For this review, take the finished solid that the model builds, in its own axes (mm). A direction names the side the tool comes from. Give positions to 0.01 mm unless a question says otherwise; leave off trailing zeros. Write each loop counter-clockwise with the first axis right and the second up, starting at its lowest first coordinate (ties: lowest second). Pieces come first, ordered by that corner, then holes.
1) For P1, Ø3, axis at y = -1, z = -4, coming from the -X side; P2, Ø2.5, axis at x = -11.5, y = 0, coming from the +Z side; P3, Ø0.8, axis at x = -8.5, z = -2.5, coming from the -Y side, all flat-tipped, find the tip position at first contact; note any pin that passes through.
2) Draft analysis for pull direction X (two halves, no side actions). For faces 5 (the face through (-1.615, 2.389, 4.751)), 6 (the face through (-13, 0, -1)), 7 (the face through (-12, 0, 0.4)), state which applies: pulls with the +X half, pulls with the -X half, needs draft (parallel to the pull), parting line crosses it, or undercut.
3) Machinability: for faces 1 (the face through (-8.4, -0.8, 2.2)), 2 (the face through (-8.5, -1.6, 0)), 3 (the face through (6.385, 2.389, -3.249)), 4 (the face through (6.5, -1, 0)), which of the approach directions +Z, -Z, +X, -X, +Y, -Y give a long, thin tool a straight path to every point of the face, cutting with its end or side? Answer none if there is none.
4) We need section D-D on y = 2.5. Give the boundary of the cut face in (x, z).
5) Wall thickness on line 1 along Z through (x, y) = (5, -0.75); line 2 along X through (y, z) = (1, 2); line 3 along X through (y, z) = (-0.5, 1.75): over which ranges is each line inside the solid? List them lowest first.
6) We need section B-B on x = -2.5. Give the boundary of the cut face in (y, z), and give its area (3 significant figures).
7) We need section A-A on y = 0. Give the boundary of the cut face in (x, z).
8) We need section C-C on z = 4. Give the boundary of the cut face in (x, y), and give its area (3 significant figures).
Autodesk Inventor part; units mm, degrees
ref_plane "YZ Plane" through (0, 0, 0) normal (1, 0, 0) x (0, 1, 0)
ref_plane "XZ Plane" through (0, 0, 0) normal (0, 1, 0) x (-1, 0, 0)
ref_plane "XY Plane" through (0, 0, 0) normal (0, 0, 1) x (1, 0, 0)
sketch "Sketch1" plane through (0, 0, 0) normal (0, 0, 1) x (1, 0, 0)
  line L0 (8, 1.6) -> (-8, 1.6)
  line L1 (-8, 1.6) -> (-8, -4.8)
  line L2 (-8, -4.8) -> (0, -4.8)
  line L3 (8, -1.6) -> (8, 1.6)
  line L4 (0, -4.8) -> (0, -1.6)
  line L5 (0, -1.6) -> (8, -1.6)
  line L6 (-11.2, 0) -> (11.2, 0) construction
  line L7 (0, -6.08) -> (0, 2.88) construction
  point P0 (0, 1.6)
  point P1 (8, 0)
  dimension "d0" = 16
  dimension "d1" = 3.2
  dimension "d2" = 6.4
extrude "Extrusion1" add sketch "Sketch1" along normal mid plane 16
sketch "Sketch2" plane through (-8, 1.6, 8) normal (0, 1, 0) x (1, 0, 0)
  line L0 (4, 12) -> (12, 12) construction
  line L1 (12, 12) -> (12, 4) construction
  line L2 (12, 4) -> (4, 4) construction
  line L3 (4, 4) -> (4, 12) construction
  line L4 (-3.2, 8) -> (19.2, 8) construction
  line L5 (8, 19.2) -> (8, -3.2) construction
  circle A0 centre (4, 12) radius 2.5
  circle A1 centre (12, 12) radius 2.5
  circle A2 centre (12, 4) radius 2.5
  circle A3 centre (4, 4) radius 2.5
  point P0 (8, 12)
  point P1 (12, 8)
  dimension "d5" = 8
  dimension "d6" = 5
extrude "Extrusion2" add sketch "Sketch2" along normal blind 1.6
sketch "Sketch4" plane through (0, 0, 0) normal (0, 1, 0) x (-1, 0, 0)
  line L0 (8, -8) -> (8, 8) construction
  line L1 (14, 0) -> (7, 0) construction
  line L2 (8, 0) -> (8, -1.6)
  line L3 (8, -1.6) -> (9, -1.6)
  line L4 (9, -1.6) -> (9, -1.4)
  line L5 (9, -1.4) -> (12.2, -1.4)
  line L6 (12.2, -1.4) -> (12.2, -1.6)
  line L7 (12.2, -1.6) -> (13, -1.6)
  line L8 (13, -1.6) -> (13, 0)
  line L9 (13, 0) -> (8, 0)
  dimension "d9" = 2.8
  dimension "d11" = 3.2
  dimension "d12" = 5
  dimension "d13" = 3.2
  dimension "d14" = 0.8
revolve "Revolution1" add sketch "Sketch4" angle 360 about axis through (-13, 0, 0) along (1, 0, 0)
sketch "Sketch5" plane through (0, 0, 0) normal (0, 1, 0) x (-1, 0, 0)
  line L0 (9, 1.6) -> (9, -1.6)
  line L1 (8, -8) -> (8, 8)
  line L2 (9, -1.6) -> (8, -3.3321)
  line L3 (9, 1.6) -> (8, 3.3321)
  dimension "d16" = 30
extrude "Extrusion3" add sketch "Sketch5" along normal mid plane 1.6
sketch "Sketch6" plane through (0, 0, 0) normal (0, 1, 0) x (-1, 0, 0)
  line L0 (13, 1.6) -> (13, -1.6) construction
  line L1 (13, -0.4) -> (10.9, -0.4)
  arc A0 (10.9, 0.4) -> (10.9, -0.4) centre (10.9, 0) ccw
  line L2 (10.9, 0.4) -> (13, 0.4)
  line L3 (13, 0.4) -> (13, -0.4)
  point P0 (13, 0)
  dimension "d19" = 0.8
  dimension "d20" = 2.5
extrude "Extrusion4" cut sketch "Sketch6" along normal through all both and the other way through all
sketch "Sketch7" plane through (0, -1.6, 8) normal (0, -1, 0) x (1, 0, 0)
  circle A0 centre (4, -4) radius 2.5 construction
  circle A1 centre (4, -12) radius 2.5 construction
  line L0 (1.5, -1.5) -> (6.5, -1.5)
  line L1 (6.5, -1.5) -> (6.5, -14.5)
  line L2 (6.5, -14.5) -> (1.5, -14.5)
  line L3 (1.5, -14.5) -> (1.5, -1.5)
  arc A2 (6.5, -5.783) -> (6.5, -10.217) centre (6.5, -8) ccw
  arc A3 (1.5, -10.217) -> (1.5, -5.783) centre (1.5, -8) ccw
extrude "Extrusion5" cut sketch "Sketch7" against normal blind 2
properties part number "LEGO Brick 4488" material "Steel"
Results list:
1. P1: stops at x = -8.47
1. P2: stops at z = 1.6
1. P3: stops at y = -0.8
2. face 5: undercut
2. face 6: pulls with the -X half
2. face 7: needs draft
3. face 1: +Z, -X, -Y
3. face 2: -X, -Y
3. face 3: +Y
3. face 4: -Y
4. outline: circle Ø5 at (-4, -4); circle Ø5 at (-4, 4); circle Ø5 at (4, -4); circle Ø5 at (4, 4)
5. line 1: z = -8 to -6.5, 6.5 to 8
5. line 2: x = -8 to 8
5. line 3: x = -8.91 to 1.5, 6.5 to 8
6. outline: (-4.8, -8) - (1.6, -8) - (1.6, -6) - (3.2, -6) - (3.2, -2) - (1.6, -2) - (1.6, 2) - (3.2, 2) - (3.2, 6) - (1.6, 6) - (1.6, 8) - (-4.8, 8) - close
6. area: 115 mm2
7. outline: (-13, -1.6) - (-12.2, -1.6) - (-12.2, -1.4) - (-9, -1.4) - (-9, -1.6) - (-8, -3.33) - (-8, -8) - (8, -8) - (8, 8) - (-8, 8) - (-8, 3.33) - (-9, 1.6) - (-9, 1.4) - (-12.2, 1.4) - (-12.2, 1.6) - (-13, 1.6) - (-13, 0.4) - (-10.9, 0.4) arc R0.4 cw to (-10.9, -0.4) - (-13, -0.4) - close; hole (1.5, -6.5) - (6.5, -6.5) - (6.5, 6.5) - (1.5, 6.5) - close
8. outline: (-8, -4.8) - (0, -4.8) - (0, -1.6) - (1.5, -1.6) - (1.5, 0.4) - (6.5, 0.4) - (6.5, -1.6) - (8, -1.6) - (8, 1.6) - (6.5, 1.6) - (6.5, 3.2) - (1.5, 3.2) - (1.5, 1.6) - (-1.5, 1.6) - (-1.5, 3.2) - (-6.5, 3.2) - (-6.5, 1.6) - (-8, 1.6) - close
8. area: 82.8 mm2
